Could you check a few things on this model? Use its own coordinates, in mm. A direction names the side the tool comes from. Give positions to 0.01 mm unless a question says otherwise; leave off trailing zeros. Loops run counter-clockwise (first coordinate to the right, second up) from the corner with the lowest first, then second, coordinate; pieces in that order, holes last. Notation, with made-up numbers: (88, 22) - (103, 22) arc R35 cw to (103, 57) - close; hole circle Ø8 at (8.5, 27). An arc over 180 degrees is marked (long way). Write each question's results on one line, items separated by ' | '. Start each with the question number.
(1) Suppose I cut it at A-A (x = -200). Please give me the cut outline in (y, z) (3 decimals), and give its area (3 significant figures).
(2) For pin 1 (5 mm diameter, centred on x = -47, z = 66.5, fed in from +Y); pin 2 (10 mm diameter, centred on x = -156, z = 76.5, fed in from -Y); pin 3 (12 mm diameter, centred on x = -179.5, y = -99.5, fed in from -Z), each with a flat end and sliding along its axis, tell me the tip position at first contact or that it passes through.
(3) If we mould it in two halves opening along Z, with no side actions, what happens to faces 1 (the face through (-245, -397, -1)), 2 (the face through (-124.08, -439.49, -10.61)), 3 (the face through (-234.86, -241.44, 193.707))? For each: released by +Z, released by -Z, zero draft, split by the parting line, or undercut.
(4) On a 3-axis mill with a long thin cutter (end or side, diameter ignored), from which of +Z, -Z, +X, -X, +Y, -Y can I reach the whole of each face in a straight line? I mean faces 4 (the face through (0, -27, 104)), 5 (the face through (-121.06, -374.04, 134.66)). Say none if no direction works.
(5) I need wall thicknesses on line 1 (X direction, y = -306.5, z = -181.5); line 2 (Z direction, x = -231, y = -205.5); line 3 (Y direction, x = -56, z = -50). Which ranges of each line are inside material? Lowest first, please.
from build123d import *

# Parameters (mm, degrees)
RACCORDO1_R                  = 10
SCHIZZO2_R                   = 10
ESTRUSIONE_ESTRUSIONE1_DEPTH = 245


with BuildPart() as part:
    # Schizzo1 → Rivoluzione1 (revolve)
    with BuildSketch(Plane.XY):
        Polygon((0, 0), (0, 42.875), (-245, 42.875), (-245, 0), (-225, 0), (-225, 22.875), (-20, 22.875), (-20, 0), align=None)
    revolve(axis=Axis((-137.660777117, -198.425, 0), (-1, 0, 0)))

    # Raccordo1
    raccordo1_edges = [part.edges().sort_by_distance(p)[0] for p in [
        (-245, -439.725, 0),
        (0, -439.725, 0),
    ]]
    fillet(raccordo1_edges, radius=RACCORDO1_R)

    # Schizzo2 → Estrusione-Estrusione1 (add)
    with BuildSketch(Plane(origin=(0, 0, 0), x_dir=(0, 0, -1), z_dir=(1, 0, 0))):
        with Locations((0, -429.725)):
            Circle(SCHIZZO2_R)
    extrude(amount=-ESTRUSIONE_ESTRUSIONE1_DEPTH)


solid = part.part
Output values:
1) outline: circle Ø482.6 at (-198.425, 0); hole circle Ø442.6 at (-198.425, 0) | area: 29,100 mm2
2) pin 1: y = 34.23 | pin 2: y = -428.89 | pin 3: z = -222.69
3) face 1: zero draft | face 2: split by the parting line | face 3: undercut
4) face 4: +Z, -Z, +X, +Y, -Y | face 5: none
5) line 1: -245 to -225, -20 to 0 | line 2: -241.2 to -198.3, 198.3 to 241.2 | line 3: -434.49 to -414, 17.15 to 37.64
